Check sheet for the modelled part. Datum: model origin and axes. Units: mm. A direction names the side the tool comes from. Give positions to 0.01 mm unless a question says otherwise; leave off trailing zeros. Order: outer loops, then holes, each group sorted by start corner. A loop starts at its lowest first (then second) coordinate and runs counter-clockwise, first axis right, second up. Notation, with made-up numbers: M -39.75,76.5 L -24.75,76.5 A20 cw -24.75,92.5 Z; hole C 28.25,-18 d11. An arc over 180 degrees is marked long. Return JSON: item names as keys, results as strings. Group by question number.
from build123d import *

# Parameters (mm, degrees)
SOCKET_1_SKETCH_W = 23.9
SOCKET_1_SKETCH_H = 6.35
SOCKET_2_SKETCH_W = 23.9
SOCKET_2_SKETCH_H = 6.35


with BuildPart() as part:
    # Filter_F1 Sketch → Filter_F1 (revolve)
    with BuildSketch(Plane.XY, mode=Mode.PRIVATE) as filter_f1_sk:
        Polygon((-44.3, 0), (-44.3, 11.988), (-22.3, 11.988), (-22.3, 13.716), (22.3, 13.716), (22.3, 11.988), (44.3, 11.988), (44.3, 0), align=None)
    revolve(filter_f1_sk.sketch.rotate(Axis((-1000, 0, 0), (1, 0, 0)), 90), axis=Axis((-1000, 0, 0), (1, 0, 0)))

    # Socket 1 Sketch → Socket 1 (revolve, cut)
    with BuildSketch(Plane.XY, mode=Mode.PRIVATE) as socket_1_sk:
        with Locations((-33.35, 3.175)):
            Rectangle(SOCKET_1_SKETCH_W, SOCKET_1_SKETCH_H)
    revolve(socket_1_sk.sketch.rotate(Axis((-1000, 0, 0), (1, 0, 0)), 90), axis=Axis((-1000, 0, 0), (1, 0, 0)), mode=Mode.SUBTRACT)

    # Socket 2 Sketch → Socket 2 (revolve, cut)
    with BuildSketch(Plane.XY, mode=Mode.PRIVATE) as socket_2_sk:
        with Locations((33.35, 3.175)):
            Rectangle(SOCKET_2_SKETCH_W, SOCKET_2_SKETCH_H)
    revolve(socket_2_sk.sketch.rotate(Axis((-1000, 0, 0), (1, 0, 0)), 90), axis=Axis((-1000, 0, 0), (1, 0, 0)), mode=Mode.SUBTRACT)


solid = part.part
1) Sectioned sample at C-C on x = -8.5. Record the boundary of the cut face in (y, z).
2) Tool access check on faces 5 (the face through (-21.4, 0, 0)), 6 (the face through (44.3, 5, 5)), 7 (the face through (33.454, -3.601, 11.434)). Record the directions out of +Z, -Z, +X, -X, +Y, -Y that give a thin tool (end or side, any length) a straight path to the whole face; none if there is none.
3) Material ranges on line 1 along Y through (x, z) = (-35, -0.5); line 2 along X through (y, z) = (9, 9.5); line 3 along X through (y, z) = (4, 3.25), recorded low to high.
4) Depth check by flat-ended pin: P1, Ø4, axis at y = -1.5, z = -2.5, coming from the -X side; P2, Ø1.5, axis at y = 11, z = -8.5, coming from the -X side; P3, Ø2, axis at x = -16, y = -10.5, coming from the -Z side. Enter the tip coordinate at first touch or a pass-through.
5) Sectioned sample at A-A on y = 0. Record the boundary of the cut face in (x, z), then the cut area to 3 significant figures.
6) Release check for a two-part mould opening along Z. For faces 1 (the face through (-33.146, -3.601, 11.434)), 2 (the face through (33.01, 3.86, -5.04)), 3 (the face through (-32.69, 3.86, -5.04)), 4 (the face through (-22.3, 12.1, -1)) record: released by +Z, released by -Z, zero draft, split by the parting line, or undercut.
7) Sectioned sample at D-D on x = 36.5. Record the boundary of the cut face in (y, z), then the cut area to 3 significant figures.
Reply:
{
 "1": {"outline": "C 0,0 d27.43"},
 "2": {"face 5": "-X", "face 6": "+Z, -Z, +X, +Y, -Y", "face 7": "+X"},
 "3": {"line 1": "-11.98 to -6.33, 6.33 to 11.98", "line 2": "-22.3 to 22.3", "line 3": "-21.4 to 21.4"},
 "4": {"P1": "x = -21.4", "P2": "x = -22.3", "P3": "z = -9.89"},
 "5": {"outline": "M -44.3,-11.99 L -22.3,-11.99 L -22.3,-13.72 L 22.3,-13.72 L 22.3,-11.99 L 44.3,-11.99 L 44.3,-6.35 L 21.4,-6.35 L 21.4,6.35 L 44.3,6.35 L 44.3,11.99 L 22.3,11.99 L 22.3,13.72 L -22.3,13.72 L -22.3,11.99 L -44.3,11.99 L -44.3,6.35 L -21.4,6.35 L -21.4,-6.35 L -44.3,-6.35 Z", "area": "1,700 mm^2"},
 "6": {"face 1": "split by the parting line", "face 2": "undercut", "face 3": "undercut", "face 4": "zero draft"},
 "7": {"outline": "C 0,0 d23.98; hole C 0,0 d12.7", "area": "325 mm^2"}
}
